Study the drawing (mm; zero at the part's minimum x, y, z) and answer. A direction names the side the tool comes from. Give positions to 0.01 mm unless a question says otherwise; leave off trailing zeros. Write each loop counter-clockwise with the first axis right and the second up, starting at its lowest first coordinate (ties: lowest second). Pieces come first, ordered by that corner, then holes.
1) Straight lines are drawn through the part: probe 1 along Y at (x, z) = (19.5, 18) (1 decimal); probe 2 along X at (y, z) = (5.5, 18.5). For each, find the intervals that lie inside material, in ascending order.
2) Find section C-C (y = 3.25). Determine the outline of the cut face in (x, z).
3) Find section A-A (z = 27). Determine the outline of the cut face in (x, y) (1 decimal).
4) Given pin 1 Ø6 at (y, z) = (23, 11.5) entering from +X; pin 2 Ø9 at (x, z) = (24.5, 10) entering from -Y; pin 3 Ø2 at (x, z) = (11, 19.5) entering from +Y (3 decimals); pin 4 Ø4.5 at (y, z) = (2, 8.5) entering from +X, each flat-ended and moving along its own axis, determine where each tip first touches the part or whether it passes through.
5) A tool of negligible diameter and unlimited length cuts with its end or side. For the marked faces 1, 2 and 3, from which of +Z, -Z, +X, -X, +Y, -Y can it reach the whole face along a straight path? Write none if from no direction.
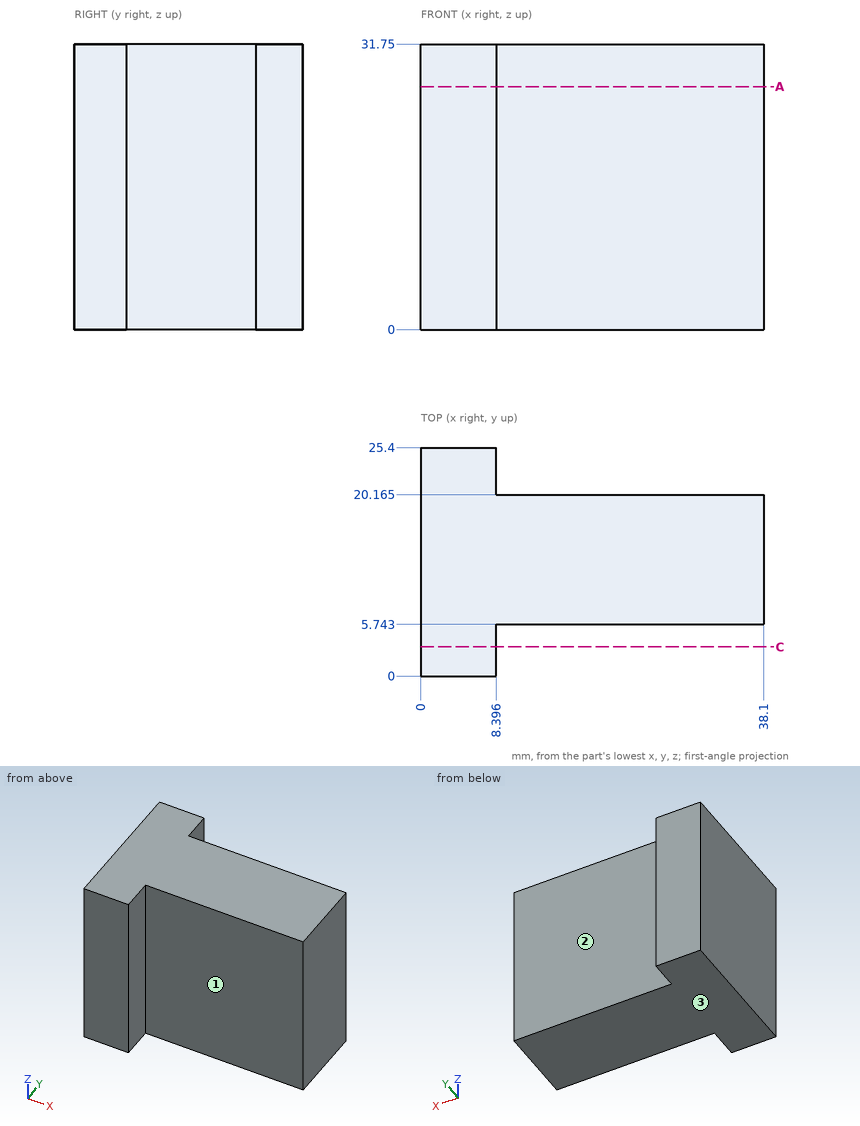
Results:
1. probe 1: y = 5.7 to 20.2
1. probe 2: x = 0 to 8.4
2. outline: (0, 0) - (8.4, 0) - (8.4, 31.75) - (0, 31.75) - close
3. outline: (0, 0) - (8.4, 0) - (8.4, 5.7) - (38.1, 5.7) - (38.1, 20.2) - (8.4, 20.2) - (8.4, 25.4) - (0, 25.4) - close
4. pin 1: stops at x = 38.1
4. pin 2: stops at y = 5.74
4. pin 3: stops at y = 20.165
4. pin 4: stops at x = 8.4
5. face 1: +Z, -Z, +X, -Y
5. face 2: +Z, -Z, +X, +Y
5. face 3: -Z, +X, -X, +Y, -Y
